```python
from build123d import *

# Parameters (mm, degrees)
SKETCH_1_R          = 2
EXTRUDE_1_DEPTH     = 5
SKETCH_2_R          = 15.5
CUT_EXTRUDE_1_DEPTH = 30


with BuildPart() as part:
    # 草图1 → 凸台-拉伸1 (new body)
    with BuildSketch(Plane.XY):
        with BuildLine():
            Line((-15.5, -25.5), (15.5, -25.5))
            ThreePointArc((15.5, -25.5), (22.571067812, -22.571067812), (25.5, -15.5))
            Line((25.5, -15.5), (25.5, 15.5))
            ThreePointArc((25.5, 15.5), (22.571067812, 22.571067812), (15.5, 25.5))
            Line((15.5, 25.5), (-15.5, 25.5))
            ThreePointArc((-15.5, 25.5), (-22.571067812, 22.571067812), (-25.5, 15.5))
            Line((-25.5, 15.5), (-25.5, -15.5))
            ThreePointArc((-25.5, -15.5), (-22.571067812, -22.571067812), (-15.5, -25.5))
        make_face()
        with Locations((-15.5, 15.5)):
            Circle(SKETCH_1_R, mode=Mode.SUBTRACT)
        with Locations((15.5, 15.5)):
            Circle(SKETCH_1_R, mode=Mode.SUBTRACT)
        with Locations((15.5, -15.5)):
            Circle(SKETCH_1_R, mode=Mode.SUBTRACT)
        with Locations((-15.5, -15.5)):
            Circle(SKETCH_1_R, mode=Mode.SUBTRACT)
    extrude(amount=EXTRUDE_1_DEPTH)

    # 草图2 → 切除-拉伸1 (cut)
    with BuildSketch(Plane.XY):
        Circle(SKETCH_2_R)
    extrude(amount=CUT_EXTRUDE_1_DEPTH, mode=Mode.SUBTRACT)


solid = part.part
```
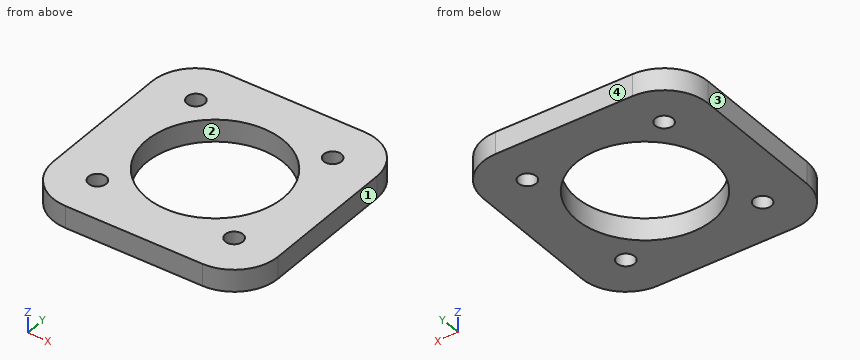
Input: part model. Units: mm. Frame: model coordinates. Face numbers are marked on the shaded views. Round coordinates to 2 decimals unless told otherwise and drop trailing zeros. Order: outer loops, then holes, each group sorted by start corner. A loop starts at its lowest first (then second) coordinate and runs counter-clockwise, first axis right, second up. Notation, with made-up numbers: (55, 37.25) - (85, 37.25) arc R17 ccw to (85, 67.25) - close; hole circle Ø6 at (-18, 11). An arc over 180 degrees is marked (long way). Answer in a Markdown table with one row per item.
Item 1: Section query C-C (z = 1.6). Return the cut outline in (x, y).
Model answer:
| item | result |
|---|---|
| outline | (-25.5, -15.5) arc R10 ccw to (-15.5, -25.5) - (15.5, -25.5) arc R10 ccw to (25.5, -15.5) - (25.5, 15.5) arc R10 ccw to (15.5, 25.5) - (-15.5, 25.5) arc R10 ccw to (-25.5, 15.5) - close; hole circle Ø4 at (-15.5, -15.5); hole circle Ø4 at (-15.5, 15.5); hole circle Ø31 at (0, 0); hole circle Ø4 at (15.5, -15.5); hole circle Ø4 at (15.5, 15.5) |
Item 2: Line query: line 1 (X direction, y = -0.5, z = 4.4); line 2 (X direction, y = -14, z = 4.5); line 3 (Y direction, x = -16.5, z = 3.55). Output: solid intervals per line, ascending.
Model answer:
| item | result |
|---|---|
| line 1 | x = -25.5 to -15.49, 15.49 to 25.5 |
| line 2 | x = -25.5 to -16.82, -14.18 to -6.65, 6.65 to 14.18, 16.82 to 25.5 |
| line 3 | y = -25.45 to -17.23, -13.77 to 13.77, 17.23 to 25.45 |
Item 3: Mould query, pull axis X, two halves, no side actions, for the marked faces 1, 2, 3 and 4. Classes: released by +X, released by -X, zero draft, split by the parting line, or undercut.
Model answer:
| item | result |
|---|---|
| face 1 | released by +X |
| face 2 | undercut |
| face 3 | released by -X |
| face 4 | zero draft |
Item 4: Section query A-A (y = 0). Return the cut outline in (x, z).
Model answer:
| item | result |
|---|---|
| outline | (-25.5, 0) - (-15.5, 0) - (-15.5, 5) - (-25.5, 5) - close; (15.5, 0) - (25.5, 0) - (25.5, 5) - (15.5, 5) - close |
Item 5: Pin query (flat end, axial travel): pin 1 (1 mm diameter, centred on y = -17.5, z = 1.5, fed in from +X); pin 2 (3.5 mm diameter, centred on x = 15.5, y = 15.5, fed in from -Z). Return the tip coordinate at first contact, or that it passes through.
Model answer:
| item | result |
|---|---|
| pin 1 | stops at x = 25.39 |
| pin 2 | passes through |
Item 6: Section query D-D (x = -20.5). Return the cut outline in (y, z).
Model answer:
| item | result |
|---|---|
| outline | (-24.16, 0) - (24.16, 0) - (24.16, 5) - (-24.16, 5) - close |
